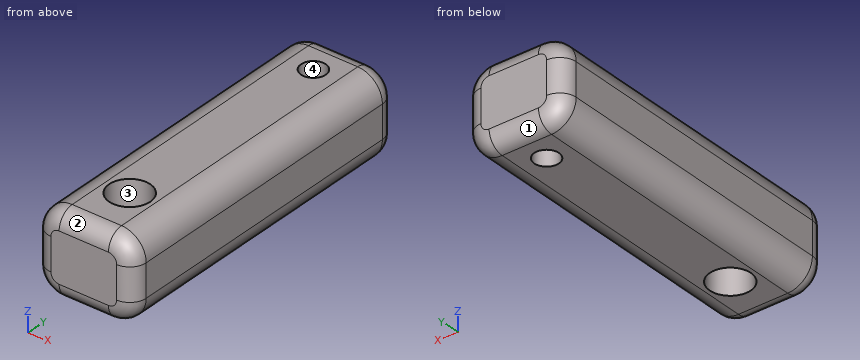
from build123d import *

# Parameters (mm, degrees)
BOSS_EXTRUDE1_DEPTH = 101.6
SKETCH2_R           = 6.35
CUT_EXTRUDE1_DEPTH  = 106.829946612
SKETCH3_R           = 3.81
CUT_EXTRUDE2_DEPTH  = 106.829946612
FILLET1_R           = 5.08
FILLET2_R           = 5.08


with BuildPart() as part:
    # Sketch1 → Boss-Extrude1 (new body)
    with BuildSketch(Plane(origin=(0, 0, 0), x_dir=(1, 0, 0), z_dir=(0, 1, 0))):
        with BuildLine():
            Line((-7.62, 12.7), (7.62, 12.7))
            ThreePointArc((7.62, 12.7), (13.008153673, 10.468153673), (15.24, 5.08))
            Line((15.24, 5.08), (15.24, -5.08))
            ThreePointArc((15.24, -5.08), (13.008153673, -10.468153673), (7.62, -12.7))
            Line((7.62, -12.7), (-7.62, -12.7))
            ThreePointArc((-7.62, -12.7), (-13.008153673, -10.468153673), (-15.24, -5.08))
            Line((-15.24, -5.08), (-15.24, 5.08))
            ThreePointArc((-15.24, 5.08), (-13.008153673, 10.468153673), (-7.62, 12.7))
        make_face()
    extrude(amount=BOSS_EXTRUDE1_DEPTH)

    # Sketch2 → Cut-Extrude1 (cut, through all)
    with BuildSketch(Plane.XY.offset(12.7)):
        with Locations((0, 17.78)):
            Circle(SKETCH2_R)
    extrude(amount=-CUT_EXTRUDE1_DEPTH, mode=Mode.SUBTRACT)

    # Sketch3 → Cut-Extrude2 (cut, through all)
    with BuildSketch(Plane.XY.offset(12.7)):
        with Locations((0, 88.9)):
            Circle(SKETCH3_R)
    extrude(amount=-CUT_EXTRUDE2_DEPTH, mode=Mode.SUBTRACT)

    # Fillet1
    fillet1_edges = [part.edges().sort_by_distance(p)[0] for p in [
        (0, 0, 12.7),
        (-13.008153673, 0, 10.468153673),
        (-15.24, 0, 0),
        (-13.008153673, 0, -10.468153673),
        (0, 0, -12.7),
        (13.008153673, 0, -10.468153673),
        (15.24, 0, 0),
        (13.008153673, 0, 10.468153673),
    ]]
    fillet(fillet1_edges, radius=FILLET1_R)

    # Fillet2
    fillet2_edges = [part.edges().sort_by_distance(p)[0] for p in [
        (13.008153673, 101.6, 10.468153673),
        (15.24, 101.6, 0),
        (13.008153673, 101.6, -10.468153673),
        (0, 101.6, -12.7),
        (-13.008153673, 101.6, -10.468153673),
        (-15.24, 101.6, 0),
        (-13.008153673, 101.6, 10.468153673),
        (0, 101.6, 12.7),
    ]]
    fillet(fillet2_edges, radius=FILLET2_R)


solid = part.part
Source: CAD feature listing. Evaluate the final solid. Frame: model axes, mm. Face numbers are marked on the shaded views. Give positions to 0.01 mm unless a question says otherwise; leave off trailing zeros. Loops run counter-clockwise (first coordinate to the right, second up) from the corner with the lowest first, then second, coordinate; pieces in that order, holes last. Notation, with made-up numbers: (71, 13) -> (119, 13) arc R28 cw to (119, 48) -> close; hole circle Ø7 at (54, 59.25). An arc over 180 degrees is marked (long way). Use a Markdown table: item, result. Add a question column.
1) Line query: line 1 along Y through (x, z) = (0, 1); line 2 along Y through (x, z) = (1, -3); line 3 along Y through (x, z) = (-10, -6.25). Output: solid intervals per line, ascending. Write a range as [from, to].
2) Pull-direction query (Y, two-part tool) for the marked faces 1, 2, 3 and 4; classes: +Y half, -Y half, draft (parallel to the pull), parting line (faces both ways), or undercut.
3) Section query C-C, the plane z = 1.25. Return the cut outline in (x, y), then the cut area to 3 significant figures.
4) Section query A-A, the plane y = 88.9. Return the cut outline in (x, z), then the cut area to 3 significant figures.
5) Section query D-D, the plane y = 17.78. Return the cut outline in (x, z), then the cut area to 3 significant figures.
6) First-contact query: pin 1 (4.5 mm diameter, centred on x = 0, y = 88.9, fed in from +Z). Flat tip, straight axial feed; report the tip coordinate or a pass-through.
7) Section query B-B, the plane x = 0. Return the cut outline in (y, z), then the cut area to 3 significant figures.
Numbers:
| question | item | result |
|---|---|---|
| 1 | line 1 | y = [0, 11.43], [24.13, 85.09], [92.71, 101.6] |
| 1 | line 2 | y = [0, 11.51], [24.05, 85.22], [92.58, 101.6] |
| 1 | line 3 | y = [0, 101.6] |
| 2 | face 1 | +Y half |
| 2 | face 2 | -Y half |
| 2 | face 3 | undercut |
| 2 | face 4 | undercut |
| 3 | outline | (-15.24, 5.08) arc R5.08 ccw to (-10.16, 0) -> (10.16, 0) arc R5.08 ccw to (15.24, 5.08) -> (15.24, 96.52) arc R5.08 ccw to (10.16, 101.6) -> (-10.16, 101.6) arc R5.08 ccw to (-15.24, 96.52) -> close; hole circle Ø12.7 at (0, 17.78); hole circle Ø7.62 at (0, 88.9) |
| 3 | area | 2,900 mm2 |
| 4 | outline | (-15.24, -5.08) arc R7.62 ccw to (-7.62, -12.7) -> (-3.81, -12.7) -> (-3.81, 12.7) -> (-7.62, 12.7) arc R7.62 ccw to (-15.24, 5.08) -> close; (3.81, -12.7) -> (7.62, -12.7) arc R7.62 ccw to (15.24, -5.08) -> (15.24, 5.08) arc R7.62 ccw to (7.62, 12.7) -> (3.81, 12.7) -> close |
| 4 | area | 531 mm2 |
| 5 | outline | (-15.24, -5.08) arc R7.62 ccw to (-7.62, -12.7) -> (-6.35, -12.7) -> (-6.35, 12.7) -> (-7.62, 12.7) arc R7.62 ccw to (-15.24, 5.08) -> close; (6.35, -12.7) -> (7.62, -12.7) arc R7.62 ccw to (15.24, -5.08) -> (15.24, 5.08) arc R7.62 ccw to (7.62, 12.7) -> (6.35, 12.7) -> close |
| 5 | area | 402 mm2 |
| 6 | pin 1 | passes through |
| 7 | outline | (0, -7.62) arc R5.08 ccw to (5.08, -12.7) -> (11.43, -12.7) -> (11.43, 12.7) -> (5.08, 12.7) arc R5.08 ccw to (0, 7.62) -> close; (24.13, -12.7) -> (85.09, -12.7) -> (85.09, 12.7) -> (24.13, 12.7) -> close; (92.71, -12.7) -> (96.52, -12.7) arc R5.08 ccw to (101.6, -7.62) -> (101.6, 7.62) arc R5.08 ccw to (96.52, 12.7) -> (92.71, 12.7) -> close |
| 7 | area | 2,040 mm2 |
